The listing builds one solid part. Answer for the finished solid, in the listing's coordinates (mm). Face numbers are marked on the shaded views. Coordinates: 2 decimals unless noted, no trailing zeros. Loops run counter-clockwise (first coordinate to the right, second up) from the corner with the lowest first, then second, coordinate; pieces in that order, holes last. Notation, with made-up numbers: (21, 2) - (78, 2) arc R25 cw to (78, 16) - close; hole circle Ø5 at (30, 55.5). An arc over 180 degrees is marked (long way). Put each result on its own line as item: value.
```python
from build123d import *

# Parameters (mm, degrees)
SKETCH_1_W      = 48
SKETCH_1_H      = 60
SKETCH_1_R      = 1.6
SKETCH_1_R_2    = 1.1
SKETCH_1_W_2    = 38
SKETCH_1_H_2    = 22
EXTRUDE_1_DEPTH = 3
FILLET_1_R      = 3
FILLET_2_R      = 3


with BuildPart() as part:
    # 草图1 → 凸台-拉伸1 (new body)
    with BuildSketch(Plane.XY):
        with Locations((0, 30)):
            Rectangle(SKETCH_1_W, SKETCH_1_H)
        with Locations((0, 6)):
            Circle(SKETCH_1_R, mode=Mode.SUBTRACT)
        with Locations((-19, 6)):
            Circle(SKETCH_1_R, mode=Mode.SUBTRACT)
        with Locations((19, 6)):
            Circle(SKETCH_1_R, mode=Mode.SUBTRACT)
        with Locations((-14, 57)):
            Circle(SKETCH_1_R_2, mode=Mode.SUBTRACT)
        with Locations((-14, 29)):
            Circle(SKETCH_1_R_2, mode=Mode.SUBTRACT)
        with Locations((14, 57)):
            Circle(SKETCH_1_R_2, mode=Mode.SUBTRACT)
        with Locations((14, 29)):
            Circle(SKETCH_1_R_2, mode=Mode.SUBTRACT)
        Polygon((-18, 10), (-3.79137849, 10), (3.79137849, 10), (18, 10), (18, 25), (-18, 25), align=None, mode=Mode.SUBTRACT)
        with Locations((0, 43)):
            Rectangle(SKETCH_1_W_2, SKETCH_1_H_2, mode=Mode.SUBTRACT)
    extrude(amount=EXTRUDE_1_DEPTH)

    # 圆角1
    fillet_1_edges = [part.edges().sort_by_distance(p)[0] for p in [
        (19, 32, 1.5),
        (19, 54, 1.5),
        (-19, 54, 1.5),
        (-19, 32, 1.5),
        (-24, 60, 1.5),
        (24, 60, 1.5),
    ]]
    fillet(fillet_1_edges, radius=FILLET_1_R)

    # 圆角2
    fillet_2_edges = [part.edges().sort_by_distance(p)[0] for p in [
        (-18, 25, 1.5),
        (-18, 10, 1.5),
        (18, 10, 1.5),
        (18, 25, 1.5),
    ]]
    fillet(fillet_2_edges, radius=FILLET_2_R)


solid = part.part
```
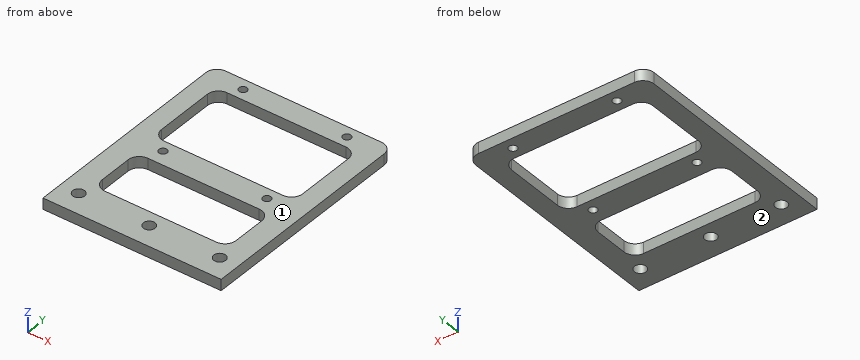
1) This flat-tipped pin is pushed along its axis until it touches: pin 1 (8 mm diameter, centred on x = 13, y = 51.5, fed in from +Z). Where does it stop, or does it pass through?
Found:
pin 1: stops at z = 3
2) The part is cut by section A-A (x = 14). Give the vertices of the cut face in (y, z), and give its area (3 significant figures).
Found:
outline: (0, 0) - (10, 0) - (10, 3) - (0, 3) - close; (25, 0) - (27.9, 0) - (27.9, 3) - (25, 3) - close; (30.1, 0) - (32, 0) - (32, 3) - (30.1, 3) - close; (54, 0) - (55.9, 0) - (55.9, 3) - (54, 3) - close; (58.1, 0) - (60, 0) - (60, 3) - (58.1, 3) - close
area: 55.8 mm^2
3) The part is cut by section D-D (z = 0.9). State how many separate pieces and enclosed holes the cut face has, and give its area (3 significant figures).
Found:
separate pieces: 1
enclosed holes: 9
area: 1,480 mm^2
4) For a pull along Z with two mould halves and no side action, classify the marked faces 1 and 2 as pulls with the +Z half, pulls with the -Z half, needs draft (parallel to the pull), parting line crosses it, or undercut.
Found:
face 1: pulls with the +Z half
face 2: pulls with the -Z half
5) The part is cut by section C-C (x = 0). Give the vertices of the cut face in (y, z).
Found:
outline: (0, 0) - (4.4, 0) - (4.4, 3) - (0, 3) - close; (7.6, 0) - (10, 0) - (10, 3) - (7.6, 3) - close; (25, 0) - (32, 0) - (32, 3) - (25, 3) - close; (54, 0) - (60, 0) - (60, 3) - (54, 3) - close
6) Straight lines are drawn through the part: L1, parallel to Y at x = 0, z = 0.9; L2, parallel to Y at x = -14, z = 1.1; L3, parallel to X at y = 13, z = 1.7. For each, find the intervals that lie inside material, in ascending order. Write a range as [from, to].
Found:
L1: y = [0, 4.4], [7.6, 10], [25, 32], [54, 60]
L2: y = [0, 10], [25, 27.9], [30.1, 32], [54, 55.9], [58.1, 60]
L3: x = [-24, -18], [18, 24]
7) The part is cut by section B-B (y = 29). Give the vertices of the cut face in (x, z).
Found:
outline: (-24, 0) - (-15.1, 0) - (-15.1, 3) - (-24, 3) - close; (-12.9, 0) - (12.9, 0) - (12.9, 3) - (-12.9, 3) - close; (15.1, 0) - (24, 0) - (24, 3) - (15.1, 3) - close
